Could you check a few things on this model? Use its own coordinates, in mm. A direction names the side the tool comes from. Round coordinates to 2 decimals unless told otherwise and drop trailing zeros. Loops run counter-clockwise (first coordinate to the right, second up) from the corner with the lowest first, then second, coordinate; pieces in that order, holes last. Notation, with made-up numbers: (79.5, -24) -> (119.5, -24) arc R28 cw to (119.5, -1) -> close; hole circle Ø4 at (57, 71.5). An arc over 180 degrees is marked (long way). One line per item, written item: value.
```python
from build123d import *

# Parameters (mm, degrees)
F0_W      = 243
F0_H      = 161
F1_DEPTH  = 19
F2_W      = 243
F2_H      = 91
F3_DEPTH  = 7.6
F4_W      = 233
F4_H      = 81
F5_DEPTH  = 3.4
F7_DEPTH  = 19
F9_DEPTH  = 7
F10_R     = 8
F12_DEPTH = 243


with BuildPart() as f1:
    # F0 (on Top) → F1 (new body)
    with BuildSketch(Plane.XY):
        with Locations((121.5, 80.5)):
            Rectangle(F0_W, F0_H)
    extrude(amount=F1_DEPTH)

    # F2 (on face) → F3 (cut)
    with BuildSketch(Plane.XY.offset(19)):
        with Locations((121.5, 115.5)):
            Rectangle(F2_W, F2_H)
    extrude(amount=-F3_DEPTH, mode=Mode.SUBTRACT)

    # F4 (on face) → F5 (cut)
    with BuildSketch(Plane.XY.offset(11.4)):
        with Locations((121.5, 115.5)):
            Rectangle(F4_W, F4_H)
    extrude(amount=-F5_DEPTH, mode=Mode.SUBTRACT)

    # F6 (on face) → F7 (cut, through all)
    with BuildSketch(Plane.XY.offset(19)):
        Polygon((12.3428886496, 0), (0, 70), (0, 0), align=None)
        Polygon((110.697450051, 40), (95.3428886496, 0), (145.3428886496, 0), (129.1186868819, 49.9329586842), align=None)
        Polygon((243, 70), (230.6571113504, 0), (243, 0), align=None)
    extrude(amount=-F7_DEPTH, mode=Mode.SUBTRACT)

    # F8 (on face) → F9 (join)
    with BuildSketch(Plane(origin=(0, 0, 0), x_dir=(1, 0, 0), z_dir=(0, 0, -1))):
        Polygon((145.3428886496, 0), (95.3428886496, 0), (110.697450051, -40), (129.1186868819, -49.9329586842), align=None)
    extrude(amount=-F9_DEPTH)

    # F10
    f10_edges = [f1.edges().sort_by_distance(p)[0] for p in [
        (0, 161, 5.7),
        (243, 161, 5.7),
        (230.657111, 0, 9.5),
        (12.342889, 0, 9.5),
        (110.69745, 40, 13),
        (129.118687, 49.932959, 13),
    ]]
    fillet(f10_edges, radius=F10_R)

    # F11 (on face) → F12 (cut, through all)
    with BuildSketch(Plane.YZ.offset(243)):
        Polygon((0, 19), (0, 10), (70, 19), align=None)
    extrude(amount=-F12_DEPTH, mode=Mode.SUBTRACT)


solid = f1.part
```
Item 1: Will these pins go through, and if not, where does the flat tip stop? pin 1 Ø2 at (x, z) = (184.5, 17) entering from +Y; pin 2 Ø14 at (x, y) = (125.5, 15.5) entering from +Z; pin 3 Ø1.5 at (x, y) = (119, 94) entering from +Z.
Output:
pin 1: stops at y = 70
pin 2: stops at z = 7
pin 3: stops at z = 8
Item 2: I need wall thicknesses on line 1 (X direction, y = 142.5, z = 9); line 2 (Y direction, x = 24, z = 8.5); line 3 (Z direction, x = 137, y = 134.5). Which ranges of each line are inside material? Lowest first, please. Write a range as from..to.
Output:
line 1: x = 0..5, 238..243
line 2: y = 0..75, 156..161
line 3: z = 0..8
Item 3: If we section it at A-A on y = 79: List the corners of the cut face in (x, z) for me, plus the area to 3 significant figures.
Output:
outline: (0, 0) -> (243, 0) -> (243, 11.4) -> (238, 11.4) -> (238, 8) -> (5, 8) -> (5, 11.4) -> (0, 11.4) -> close
area: 1,980 mm²
Item 4: For faces 1 (the face through (117, 43.4, 11.5)), 2 (the face through (123, 0, 5)), which set-ups out of +Z, -Z, +X, -X, +Y, -Y let a thin tool reach every point of the face, with its end or its side?
Output:
face 1: +Z, -Y
face 2: +Z, -Z, +X, -X, -Y
Item 5: If we section it at B-B on x = 42: List the corners of the cut face in (y, z) for me, plus the area to 3 significant figures.
Output:
outline: (0, 0) -> (161, 0) -> (161, 11.4) -> (156, 11.4) -> (156, 8) -> (75, 8) -> (75, 11.4) -> (70, 11.4) -> (70, 19) -> (0, 10) -> close
area: 1,780 mm²
Item 6: If we section it at D-D on y = 56.5: List the corners of the cut face in (x, z) for me, plus the area to 3 significant figures.
Output:
outline: (2.38, 0) -> (240.62, 0) -> (240.62, 17.26) -> (2.38, 17.26) -> close
area: 4,110 mm²
Item 7: If we mould it in two halves opening along X, with no side actions, what happens to faces 3 (the face through (84.9, 156.2, 11.4)), 4 (the face through (243, 111, 6)), 5 (the face through (127.36, 45.8, 11.44)), 6 (the face through (120, 116, 8))? For each: released by +X, released by -X, zero draft, split by the parting line, or undercut.
Output:
face 3: zero draft
face 4: released by +X
face 5: undercut
face 6: undercut
Item 8: If we section it at C-C on y = 32: List the corners of the cut face in (x, z) for me, plus the area to 3 significant figures.
Output:
outline: (6.7, 0) -> (236.3, 0) -> (236.3, 14.11) -> (134.95, 14.11) -> (134.95, 7) -> (107.63, 7) -> (107.63, 14.11) -> (6.7, 14.11) -> close
area: 3,050 mm²
